Design review of the part built by this model. Coordinates are the model's own, in mm. Face numbers are marked on the shaded views. A direction names the side the tool comes from. Give positions to 0.01 mm unless a question says otherwise; leave off trailing zeros. Write each loop counter-clockwise with the first axis right and the second up, starting at its lowest first coordinate (ties: lowest second). Pieces come first, ordered by that corner, then holes. Notation, with made-up numbers: M 1.5,-40 L 45.5,-40 A21 cw 45.5,-18 Z; hole C 19.5,55 d6. An arc over 180 degrees is marked long. Answer in a Markdown table with one row per item.
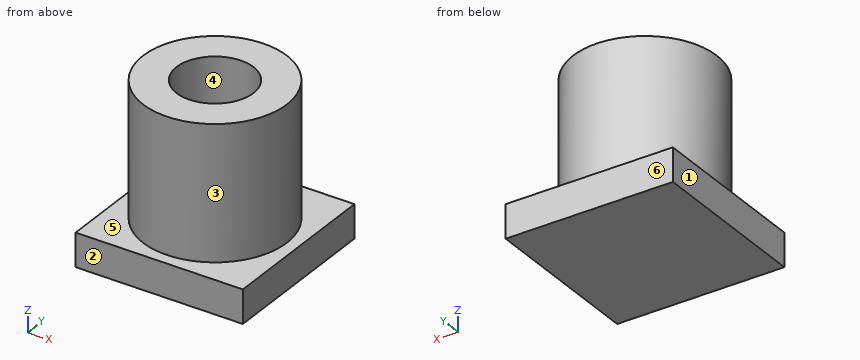
Autodesk Fusion 360 part; units mm, degrees
sketch "Skizze1" plane through (0, 0, 0) normal (0, 0, 1) x (1, 0, 0)
  line L0 (-4, 4) -> (4, 4)
  line L1 (4, 4) -> (4, -4)
  line L2 (4, -4) -> (-4, -4)
  line L3 (-4, -4) -> (-4, 4)
  line L4 (-4, 4) -> (4, -4) construction
  line L5 (4, 4) -> (-4, -4) construction
  dimension "d1" = 8
  dimension "d2" = 8
extrude "Extrusion1" add sketch "Skizze1" along normal blind 2
sketch "Skizze2" plane through (0, 0, 2) normal (0, 0, 1) x (-1, 0, 0)
  line L0 (4, 4) -> (-4, 4)
  line L1 (-4, 4) -> (-4, -4)
  line L2 (-4, -4) -> (4, -4)
  line L3 (4, -4) -> (4, 4)
  circle A0 centre (0, 0) radius 2.3
  circle A1 centre (0, 0) radius 3.3
  dimension "d5" = 4.6
  dimension "d6" = 6.6
extrude "Extrusion2" add sketch "Skizze2" along normal blind 8 contours A1
extrude "Extrusion3" add 1 faces at (0.6334, 0.4319, 2) along direction (0, 0, 1) blind 2
extrude "Extrusion4" add 1 faces at (1.3333, -4, 0.6667) along direction (0, -1, 0) blind 1
extrude "Extrusion5" add 1 faces at (4, 1, 0.6667) along direction (1, 0, 0) blind 1
extrude "Extrusion6" add 1 faces at (2, 4, 1.3333) along direction (0, 1, 0) blind 1
extrude "Extrusion7" add 1 faces at (-4, 1.6667, 0.6667) along direction (-1, 0, 0) blind 1
move_face "Flächen versetzen1" offset 1 1 faces at (-3.2959, 0.1645, 7.3333)
1) Add section C-C (z = 5.75). Write out the cut boundary in (x, y).
Geometry says:
| item | result |
|---|---|
| outline | C 0,0 d8.6; hole C 0,0 d4.6 |
2) Add section D-D (x = 3.5). Write out the cut boundary in (y, z), and give its area (3 significant figures).
Geometry says:
| item | result |
|---|---|
| outline | M -5,0 L 5,0 L 5,2 L 2.5,2 L 2.5,10 L -2.5,10 L -2.5,2 L -5,2 Z |
| area | 60.0 mm^2 |
3) The part is to be moulded in two halves that separate along Y. For the marked faces 1, 2, 3 and 4, say which applies: released by +Y, released by -Y, zero draft, split by the parting line, or undercut.
Geometry says:
| item | result |
|---|---|
| face 1 | zero draft |
| face 2 | released by -Y |
| face 3 | split by the parting line |
| face 4 | undercut |
4) Add section A-A (y = 0). Write out the cut boundary in (x, z), and give its area (3 significant figures).
Geometry says:
| item | result |
|---|---|
| outline | M -5,0 L 5,0 L 5,2 L 4.3,2 L 4.3,10 L 2.3,10 L 2.3,4 L -2.3,4 L -2.3,10 L -4.3,10 L -4.3,2 L -5,2 Z |
| area | 61.2 mm^2 |
5) For the marked faces 5 and 6, list the 3-axis set-ups (+Z, -Z, +X, -X, +Y, -Y) from which the entire face can be reached by the end or side of a thin tool; tool diameter is ignored.
Geometry says:
| item | result |
|---|---|
| face 5 | +Z |
| face 6 | +Z, -Z, +X, -X, +Y |
6) Insertion check: P1, Ø3, axis at x = 3, z = 4, coming from the -Y side; P2, Ø5, axis at x = -3, z = 5, coming from the -Y side; P3, Ø6, axis at y = 0, z = 7, coming from the +X side. Each pin has a flat end and moves straight along its axis. Give the tip position at first contact, or say it passes through.
Geometry says:
| item | result |
|---|---|
| P1 | y = -4.03 |
| P2 | y = -4.27 |
| P3 | x = 4.3 |
7) To check wall thickness, follow probe 1 along Y at (x, z) = (0, 8.05); probe 2 along Z at (x, y) = (0, 1); probe 3 along X at (y, z) = (-0.75, 4.25). State the ranges of each line that lie inside material, in increasing order. Write a range as [from, to].
Geometry says:
| item | result |
|---|---|
| probe 1 | [-4.3, -2.3], [2.3, 4.3] |
| probe 2 | [0, 4] |
| probe 3 | [-4.23, -2.17], [2.17, 4.23] |
